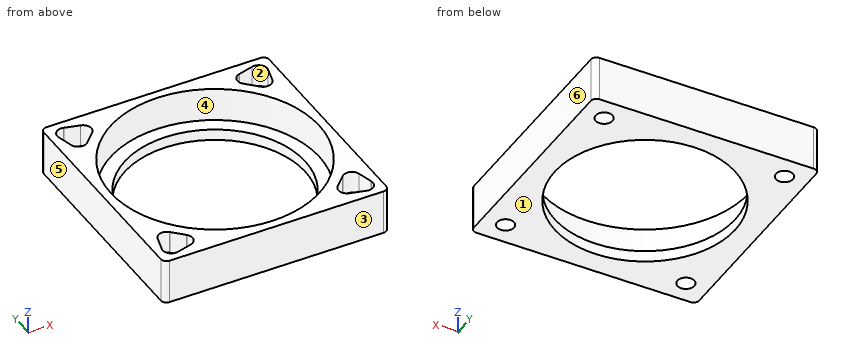
from build123d import *

# Parameters (mm, degrees)
SKETCH_W        = 40
SKETCH_H        = 40
SKETCH_R        = 16
PAD_DEPTH       = 8
SKETCH005_R     = 1.5
POCKET003_DEPTH = 8.001
POCKET_DEPTH    = 4
SKETCH006_R     = 18.5
POCKET004_DEPTH = 6
FILLET_R        = 1


with BuildPart() as part:
    # Sketch → Pad (new body)
    with BuildSketch(Plane.XY):
        Rectangle(SKETCH_W, SKETCH_H)
        Circle(SKETCH_R, mode=Mode.SUBTRACT)
    extrude(amount=PAD_DEPTH)

    # Sketch005 (on Face6 of Pad) → Pocket003 (cut, through all)
    with BuildSketch(Plane(origin=(0, 0, 0), x_dir=(1, 0, 0), z_dir=(0, 0, -1))):
        with Locations((-16, 16)):
            Circle(SKETCH005_R)
        with Locations((16, 16)):
            Circle(SKETCH005_R)
        with Locations((-16, -16)):
            Circle(SKETCH005_R)
        with Locations((16, -16)):
            Circle(SKETCH005_R)
    extrude(amount=-POCKET003_DEPTH, mode=Mode.SUBTRACT)

    # Sketch004 (on Face5 of Pocket003) → Pocket (cut)
    with BuildSketch(Plane.XY.offset(8)):
        with BuildLine():
            Line((13.434683, 15.312625), (15.312625, 13.434683))
            Line((15.312625, 13.434683), (15.35345, 13.393859))
            ThreePointArc((15.35345, 13.393859), (16.802339, 13.00563), (17.862999, 14.06629))
            Line((17.877942, 14.122058), (17.862999, 14.06629))
            Line((17.877942, 14.122058), (18.565317, 16.687375))
            Line((18.565317, 16.687375), (18.58026, 16.743142))
            ThreePointArc((18.58026, 16.743142), (18.192031, 18.192031), (16.743142, 18.58026))
            Line((16.687375, 18.565317), (16.743142, 18.58026))
            Line((16.687375, 18.565317), (14.122058, 17.877942))
            Line((14.122058, 17.877942), (14.06629, 17.862999))
            ThreePointArc((14.06629, 17.862999), (13.00563, 16.802339), (13.393859, 15.35345))
            Line((13.434683, 15.312625), (13.393859, 15.35345))
        make_face()
        with BuildLine():
            Line((14.122058, -17.877942), (16.687375, -18.565317))
            Line((16.687375, -18.565317), (16.743142, -18.58026))
            ThreePointArc((16.743142, -18.58026), (18.192031, -18.192031), (18.58026, -16.743142))
            Line((18.565317, -16.687375), (18.58026, -16.743142))
            Line((18.565317, -16.687375), (17.877942, -14.122058))
            Line((17.877942, -14.122058), (17.862999, -14.06629))
            ThreePointArc((17.862999, -14.06629), (16.802339, -13.00563), (15.35345, -13.393859))
            Line((15.312625, -13.434683), (15.35345, -13.393859))
            Line((15.312625, -13.434683), (13.434683, -15.312625))
            Line((13.434683, -15.312625), (13.393859, -15.35345))
            ThreePointArc((13.393859, -15.35345), (13.00563, -16.802339), (14.06629, -17.862999))
            Line((14.122058, -17.877942), (14.06629, -17.862999))
        make_face()
        with BuildLine():
            Line((-14.122058, 17.877942), (-16.687375, 18.565317))
            Line((-16.687375, 18.565317), (-16.743142, 18.58026))
            ThreePointArc((-16.743142, 18.58026), (-18.192031, 18.192031), (-18.58026, 16.743142))
            Line((-18.565317, 16.687375), (-18.58026, 16.743142))
            Line((-18.565317, 16.687375), (-17.877942, 14.122058))
            Line((-17.877942, 14.122058), (-17.862999, 14.06629))
            ThreePointArc((-17.862999, 14.06629), (-16.802339, 13.00563), (-15.35345, 13.393859))
            Line((-15.312625, 13.434683), (-15.35345, 13.393859))
            Line((-15.312625, 13.434683), (-13.434683, 15.312625))
            Line((-13.434683, 15.312625), (-13.393859, 15.35345))
            ThreePointArc((-13.393859, 15.35345), (-13.00563, 16.802339), (-14.06629, 17.862999))
            Line((-14.122058, 17.877942), (-14.06629, 17.862999))
        make_face()
        with BuildLine():
            Line((-13.434683, -15.312625), (-15.312625, -13.434683))
            Line((-15.312625, -13.434683), (-15.35345, -13.393859))
            ThreePointArc((-15.35345, -13.393859), (-16.802339, -13.00563), (-17.862999, -14.06629))
            Line((-17.877942, -14.122058), (-17.862999, -14.06629))
            Line((-17.877942, -14.122058), (-18.565317, -16.687375))
            Line((-18.565317, -16.687375), (-18.58026, -16.743142))
            ThreePointArc((-18.58026, -16.743142), (-18.192031, -18.192031), (-16.743142, -18.58026))
            Line((-16.687375, -18.565317), (-16.743142, -18.58026))
            Line((-16.687375, -18.565317), (-14.122058, -17.877942))
            Line((-14.122058, -17.877942), (-14.06629, -17.862999))
            ThreePointArc((-14.06629, -17.862999), (-13.00563, -16.802339), (-13.393859, -15.35345))
            Line((-13.434683, -15.312625), (-13.393859, -15.35345))
        make_face()
    extrude(amount=-POCKET_DEPTH, mode=Mode.SUBTRACT)

    # Sketch006 (on Face5 of Pocket) → Pocket004 (cut)
    with BuildSketch(Plane.XY.offset(8)):
        Circle(SKETCH006_R)
    extrude(amount=-POCKET004_DEPTH, mode=Mode.SUBTRACT)

    # Fillet
    fillet_edges = [part.edges().sort_by_distance(p)[0] for p in [
        (-20, -20, 4),
        (-20, 20, 4),
        (20, -20, 4),
        (20, 20, 4),
    ]]
    fillet(fillet_edges, radius=FILLET_R)


solid = part.part
Verification items for the finished model (mm, model axes). Face numbers are marked on the shaded views. A direction names the side the tool comes from. Round coordinates to 2 decimals unless told otherwise and drop trailing zeros. Write each loop counter-clockwise with the first axis right and the second up, starting at its lowest first coordinate (ties: lowest second). Pieces come first, ordered by that corner, then holes.
(1) Mould release check, pull along X, two halves, no side actions. Record for the marked faces 3, 4, 5 and 6: pulls with the +X half, pulls with the -X half, needs draft (parallel to the pull), parting line crosses it, or undercut.
Returned:
face 3: needs draft
face 4: undercut
face 5: pulls with the -X half
face 6: pulls with the +X half
(2) Depth check by flat-ended pin: pin 1 Ø4 at (x, y) = (-16, 16) entering from -Z; pin 2 Ø3 at (x, y) = (-15, 16.5) entering from +Z; pin 3 Ø4 at (x, y) = (4, -14) entering from +Z. Enter the tip coordinate at first touch or a pass-through.
Returned:
pin 1: stops at z = 0
pin 2: stops at z = 4
pin 3: stops at z = 2
(3) Section check A-A (x = 0). Enter the section's corners in (y, z), plus the area to 3 significant figures.
Returned:
outline: (-20, 0) - (-16, 0) - (-16, 2) - (-18.5, 2) - (-18.5, 8) - (-20, 8) - close; (16, 0) - (20, 0) - (20, 8) - (18.5, 8) - (18.5, 2) - (16, 2) - close
area: 34.0 mm2
(4) Material ranges on line 1 (X direction, y = 0, z = 0.55); line 2 (Y direction, x = 16, z = 3); line 3 (X direction, y = 14.5, z = 5.5), recorded low to high.
Returned:
line 1: x = -20 to -16, 16 to 20
line 2: y = -20 to -17.5, -14.5 to -9.29, 9.29 to 14.5, 17.5 to 20
line 3: x = -20 to -17.98, -14.25 to -11.49, 11.49 to 14.25, 17.98 to 20
(5) Access from +Z, -Z, +X, -X, +Y, -Y to the whole of each face (thin tool, end or side, straight path). Record for the marked faces 1 and 2.
Returned:
face 1: -Z, +X, -X, +Y, -Y
face 2: +Z
(6) Section check C-C (z = 6.5). Give the number of separate pieces and of enclosed holes in the cut face, plus the area to 3 significant figures.
Returned:
separate pieces: 1
enclosed holes: 5
area: 432 mm2
